Autodesk Inventor part; units mm, degrees
ref_plane "YZ Plane" through (0, 0, 0) normal (1, 0, 0) x (0, 1, 0)
ref_plane "XZ Plane" through (0, 0, 0) normal (0, 1, 0) x (-1, 0, 0)
ref_plane "XY Plane" through (0, 0, 0) normal (0, 0, 1) x (1, 0, 0)
sketch "スケッチ1" plane through (0, 0, 0) normal (0, 0, 1) x (1, 0, 0)
  line L0 (0, 0) -> (-15, 0)
  line L1 (-15, 0) -> (-15, 20)
  line L2 (-15, 20) -> (0, 20)
  line L3 (0, 20) -> (0, 0)
  line L4 (0, 0) -> (0, 43.6966) construction
  line L5 (-15, 12.5) -> (-20, 12.5)
  line L6 (-20, 12.5) -> (-20, 0)
  line L7 (-30, 0) -> (-30, 12.5)
  line L8 (-30, 0) -> (-20, 0)
  line L9 (23.8812, 0) -> (-169.724, 0) construction
  line L10 (-45, 0) -> (-45, 12.5)
  line L11 (-45, 0) -> (-35, 0)
  line L12 (-35, 12.5) -> (-35, 0)
  line L13 (-30, 12.5) -> (-35, 12.5)
  line L14 (-60, 0) -> (-60, 12.5)
  line L15 (-60, 0) -> (-50, 0)
  line L16 (-50, 12.5) -> (-50, 0)
  line L17 (-45, 12.5) -> (-50, 12.5)
  line L18 (-75, 0) -> (-75, 12.5)
  line L19 (-75, 0) -> (-65, 0)
  line L20 (-65, 12.5) -> (-65, 0)
  line L21 (-60, 12.5) -> (-65, 12.5)
  line L22 (-75, 0) -> (-80, 0)
  line L23 (-80, 0) -> (-80, 20)
  line L24 (-80, 20) -> (-75, 20)
  line L25 (-75, 20) -> (-75, 0)
  line L26 (-75, 20) -> (-15, 20)
  line L27 (-75, 0) -> (-80, 5)
  line L28 (-75, 0) -> (-67.9289, 0) construction
  line L29 (0, 5) -> (-5, 0)
  line L30 (-40, 30.9864) -> (-40, -18.8288) construction
  line L31 (-42.5, 17.5) -> (-37.5, 17.5)
  line L32 (-37.5, 17.5) -> (-37.5, 5)
  line L33 (-37.5, 5) -> (-42.5, 5)
  line L34 (-42.5, 5) -> (-42.5, 17.5)
  line L35 (-42.5, 17.5) -> (-37.5, 5) construction
  line L36 (-37.5, 17.5) -> (-42.5, 5) construction
  line L37 (-57.5, 5) -> (-57.5, 17.5)
  line L38 (-52.5, 17.5) -> (-52.5, 5)
  line L39 (-52.5, 5) -> (-57.5, 5)
  line L40 (-72.5, 5) -> (-72.5, 17.5)
  line L41 (-67.5, 17.5) -> (-67.5, 5)
  line L42 (-67.5, 5) -> (-72.5, 5)
  line L43 (-27.5, 5) -> (-27.5, 17.5)
  line L44 (-22.5, 17.5) -> (-22.5, 5)
  line L45 (-22.5, 5) -> (-27.5, 5)
  line L46 (-42.5, 5) -> (-42.5, 17.5)
  line L47 (-37.5, 17.5) -> (-37.5, 5)
  line L48 (-37.5, 5) -> (-42.5, 5)
  line L49 (-57.5, 5) -> (-57.5, 17.5)
  line L50 (-52.5, 17.5) -> (-52.5, 5)
  line L51 (-52.5, 5) -> (-57.5, 5)
  line L52 (-12.5, 5) -> (-12.5, 17.5)
  line L53 (-7.5, 17.5) -> (-7.5, 5)
  line L54 (-7.5, 5) -> (-12.5, 5)
  line L55 (-27.5, 5) -> (-27.5, 17.5)
  line L56 (-22.5, 17.5) -> (-22.5, 5)
  line L57 (-22.5, 5) -> (-27.5, 5)
  line L58 (-42.5, 5) -> (-42.5, 17.5)
  line L59 (-37.5, 17.5) -> (-37.5, 5)
  line L60 (-37.5, 5) -> (-42.5, 5)
  line L61 (-72.5, 17.5) -> (-7.5, 17.5)
  line L62 (-72.5, 15) -> (-7.5, 15)
  point P0 (-40, 11.25)
  point P1 (-67.5, 15)
  point P2 (-57.5, 15)
  point P3 (-52.5, 15)
  point P4 (-42.5, 15)
  point P5 (-37.5, 15)
  point P6 (-27.5, 15)
  point P7 (-22.5, 15)
  point P8 (-12.5, 15)
  dimension "d4" = 15
  dimension "d5" = 20
  dimension "d6" = 5
  dimension "d7" = 10
  dimension "d8" = 7.5
  dimension "d9" = 15
  dimension "d10" = 5
  dimension "d11" = 135
  dimension "d12" = 5
  dimension "d13" = 135
  dimension "d17" = 12.5
  dimension "d18" = 5
  dimension "d19" = 5
  dimension "d22" = 15
  dimension "d25" = 15
  dimension "d28" = 2.5
extrude "押し出し1" add sketch "スケッチ1" along normal blind 7.5 contours L62 L44 L61 L1 | L1 L61 L52 L62 | L62 L43 L61 L44 | L44 L45 L43 L62 | L62 L53 L54 L52 | L52 L61 L53 L62 | L62 L32 L61 L43 | L62 L34 L31 L32 | L32 L33 L34 L62 | L62 L38 L61 L34 | L62 L37 L61 L38 | L38 L39 L37 L62 | L62 L41 L61 L37 | L62 L40 L61 L41 | L41 L42 L40 L62
mirror "ミラー1" about plane through (-40, 11.25, 0) normal (0, 0, -1) of "押し出し1"
properties part number "chamber"
The listing builds one solid part. Answer for the finished solid, in the listing's coordinates (mm). A direction names the side the tool comes from. Coordinates: 2 decimals unless noted, no trailing zeros. Loops run counter-clockwise (first coordinate to the right, second up) from the corner with the lowest first, then second, coordinate; pieces in that order, holes last. Notation, with made-up numbers: (28, 0) -> (38, 0) arc R6 ccw to (38, 9) -> close; hole circle Ø10 at (56, 20.25). An arc over 180 degrees is marked (long way). Use one line per item in the form item = value. Start each with the question number.
Item 1: The part is cut by section A-A on y = 14.25. Determine the outline of the cut face in (x, z), then the cut area to 3 significant figures.
Item 2: The mould has two halves that part along X. Classify faces 3 (the face through (-63, 15, 0)), 4 (the face through (-70, 5, 0)), 5 (the face through (-37.5, 10, 0)), 6 (the face through (-72.5, 11, 0)): released by +X, released by -X, zero draft, split by the parting line, or undercut.
Item 3: The part is cut by section B-B on z = 3. Determine the outline of the cut face in (x, y), then the cut area to 4 significant figures.
Item 4: Consider L1, parallel to X at y = 6.25, z = -6; L2, parallel to Y at x = -64.5, z = -6.25. Determine where each line is inside the solid, lowest interval first. Write a range as [from, to].
Item 5: The part is cut by section C-C on x = -64. Determine the outline of the cut face in (y, z), then the cut area to 3 significant figures.
Item 6: A tool of negligible diameter and unlimited length cuts with its end or side. For faces 1 (the face through (-57.5, 10, 0)), 2 (the face through (-25, 5, 0)), from which of +Z, -Z, +X, -X, +Y, -Y can it reach the whole face along a straight path? Write none if from no direction.
Item 7: A flat-ended cylindrical pin translates along its axis: pin 1 Ø3 at (x, z) = (-60.5, -1.5) entering from -Y. Find the tip coordinate at first contact, or state that the pin passes through.
Answer key:
q1.outline = (-72.5, -7.5) -> (-67.5, -7.5) -> (-67.5, 7.5) -> (-72.5, 7.5) -> close; (-57.5, -7.5) -> (-52.5, -7.5) -> (-52.5, 7.5) -> (-57.5, 7.5) -> close; (-42.5, -7.5) -> (-37.5, -7.5) -> (-37.5, 7.5) -> (-42.5, 7.5) -> close; (-27.5, -7.5) -> (-22.5, -7.5) -> (-22.5, 7.5) -> (-27.5, 7.5) -> close; (-12.5, -7.5) -> (-7.5, -7.5) -> (-7.5, 7.5) -> (-12.5, 7.5) -> close
q1.area = 375 mm2
q2.face_3 = undercut
q2.face_4 = zero draft
q2.face_5 = undercut
q2.face_6 = released by -X
q3.outline = (-72.5, 5) -> (-67.5, 5) -> (-67.5, 15) -> (-57.5, 15) -> (-57.5, 5) -> (-52.5, 5) -> (-52.5, 15) -> (-42.5, 15) -> (-42.5, 5) -> (-37.5, 5) -> (-37.5, 15) -> (-27.5, 15) -> (-27.5, 5) -> (-22.5, 5) -> (-22.5, 15) -> (-12.5, 15) -> (-12.5, 5) -> (-7.5, 5) -> (-7.5, 17.5) -> (-72.5, 17.5) -> close
q3.area = 412.5 mm2
q4.L1 = [-72.5, -67.5], [-57.5, -52.5], [-42.5, -37.5], [-27.5, -22.5], [-12.5, -7.5]
q4.L2 = [15, 17.5]
q5.outline = (15, -7.5) -> (17.5, -7.5) -> (17.5, 7.5) -> (15, 7.5) -> close
q5.area = 37.5 mm2
q6.face_1 = +Z, -Z, -Y
q6.face_2 = +Z, -Z, +X, -X, -Y
q7.pin_1 = 15
